```python
from build123d import *

# Parameters (mm, degrees)
SKETCH1_W           = 32.66
SKETCH1_H           = 5.66
BOSS_EXTRUDE1_DEPTH = 66.3
BOSS_EXTRUDE3_DEPTH = 7
F_3DSKETCH2_R       = 3.086177745
F_3DSKETCH2_R_2     = 2.932442158
CUT_EXTRUDE1_DEPTH  = 0.1


with BuildPart() as part:
    # Sketch1 → Boss-Extrude1 (new body)
    with BuildSketch(Plane.XY):
        with Locations((-4.344198718, -1.121650641)):
            Rectangle(SKETCH1_W, SKETCH1_H)
    extrude(amount=BOSS_EXTRUDE1_DEPTH)


with BuildPart() as boss_extrude3_tool:
    # 3DSketch1 → Boss-Extrude3 (new, along a direction that is not the sketch's normal)
    with BuildSketch(Plane(origin=(-15.174198718, -1.178373292, 66.3), x_dir=(0.9999872662359682, 0.005046520163970641, -3.866762069669127e-07), z_dir=(-4.534508681961708e-07, 1.3230678756319878e-05, -0.9999999999123718))):
        Polygon((0, 0), (7.99989813, 0.040372161), (8.000402782, -0.059626565), (0.000504652, -0.099998727), align=None)
        Polygon((13.729853573, 0.063545778), (21.729762739, 0.101958696), (21.730277042, 0), (13.730369262, -0.038412192), align=None)
    extrude(amount=-BOSS_EXTRUDE3_DEPTH, dir=(0, 0, -1))


with BuildPart() as part_1:
    add(part.part)


with BuildPart() as part_2:
    # Boss-Extrude3: joined with boss_extrude3_tool
    add(part_1.part.fuse(boss_extrude3_tool.part, tol=0.00001))

    # 3DSketch2 → Cut-Extrude1 (cut)
    # profile 1 of 2: a face of its own
    with BuildSketch(Plane(origin=(-14.000400956, -3.951650641, 62.768913979), x_dir=(0.9972629704452686, 0, 0.07393624130749163), z_dir=(0, 1, 0))):
        with Locations(Location((2.573415081, 0, 0), (0, 0, 94.240103716))):
            Circle(F_3DSKETCH2_R)
        with Locations(Location((2.573415081, 0, 0), (0, 0, 94.240103716))):
            Circle(F_3DSKETCH2_R_2, mode=Mode.SUBTRACT)
    # profile 2 of 2: a face of its own
    with BuildSketch(Plane(origin=(-14.000400956, -3.951650641, 62.768913979), x_dir=(0.9972629704452686, 0, 0.07393624130749163), z_dir=(0, 1, 0))):
        Polygon((0, 0), (5.118694666, 0.379495735), (5.146830162, 0), (0.028135496, -0.379495735), align=None)
    extrude(amount=CUT_EXTRUDE1_DEPTH, mode=Mode.SUBTRACT)


solid = part_2.part
```
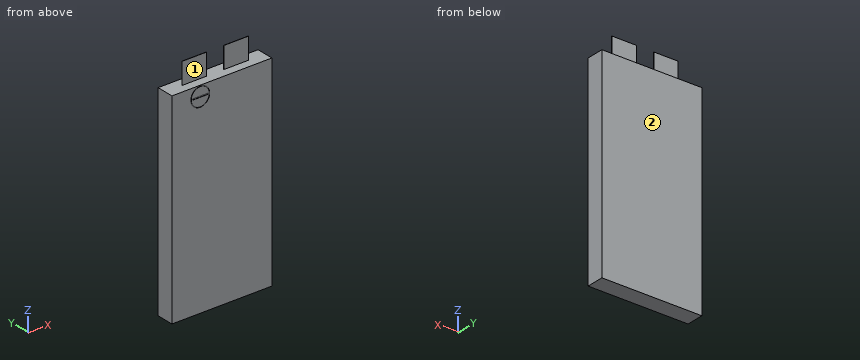
Here's how the part is built. I have some questions about the finished solid (model axes, mm). Face numbers are marked on the shaded views. A direction names the side the tool comes from. Coordinates: 2 decimals unless noted, no trailing zeros. Order: outer loops, then holes, each group sorted by start corner. A loop starts at its lowest first (then second) coordinate and runs counter-clockwise, first axis right, second up.
1) Imagine slicing it at B-B on x = 4. List the corners of the cut face in (y, z) for me.
2) Will these pins go through, and if not, where does the flat tip stop? pin 1 (3.5 mm diameter, centred on x = 1.5, z = 68.5, fed in from -Y); pin 2 (7.5 mm diameter, centred on x = 3.5, z = 70, fed in from +Y).
3) I need wall thicknesses on line 1 (Z direction, x = -10, y = -1.5). Which ranges of the line are inside material? Lowest first, please.
4) Which directions (+Z, -Z, +X, -X, +Y, -Y) give clear straight access to the entire face, cutting with the end or side of a thin tool? Please do the marked faces 1 and 2.
5) Imagine slicing it at A-A on y = 0.2. List the corners of the cut face in (x, z) for me, and give its area (3 significant figures).
6) Imagine slicing it at C-C on x = 8.5. List the corners of the cut face in (y, z) for me, and give its area (3 significant figures).
Response values:
1. outline: (-3.95, 0) - (1.71, 0) - (1.71, 66.3) - (-1.07, 66.3) - (-1.07, 73.3) - (-1.17, 73.3) - (-1.17, 66.3) - (-3.95, 66.3) - close
2. pin 1: stops at y = -1.17
2. pin 2: stops at y = 1.71
3. line 1: z = 0 to 66.3
4. face 1: +Z, +X, -X, -Y
4. face 2: +Z, -Z, +X, -X, +Y
5. outline: (-20.67, 0) - (11.99, 0) - (11.99, 66.3) - (-20.67, 66.3) - close
5. area: 2,170 mm2
6. outline: (-3.95, 0) - (1.71, 0) - (1.71, 66.3) - (-3.95, 66.3) - close
6. area: 375 mm2
